Source: CAD feature listing. Evaluate the final solid. Frame: model axes, mm. A direction names the side the tool comes from. Give positions to 0.01 mm unless a question says otherwise; leave off trailing zeros. Write each loop counter-clockwise with the first axis right and the second up, starting at its lowest first coordinate (ties: lowest second). Pieces come first, ordered by that corner, then holes. Notation, with made-up numbers: (-28, 63.25) -> (20, 63.25) arc R29 cw to (20, 85.25) -> close; hole circle Ø1 at (89.25, -7.75). An arc over 180 degrees is marked (long way). Answer as a JSON object with one key per item and string values. Group by question number.
Item 1: Pull-direction query (X, two-part tool) for faces 1 (the face through (18.01, 9.86, -72.15)), 2 (the face through (27, 5, -103)), 3 (the face through (9, 10, 0)); classes: pulls with the +X half, pulls with the -X half, needs draft (parallel to the pull), parting line crosses it, or undercut.
Item 2: Section query B-B on z = -28. Return the cut outline in (x, y), plus the area to 3 significant figures.
Item 3: Section query D-D on z = -97. Return the cut outline in (x, y).
Item 4: Section query A-A on y = 8. Return the cut outline in (x, z).
Item 5: Ray query, probe 1 along X at (y, z) = (16, -26); probe 2 along Z at (x, y) = (31, 5.5); probe 3 along Z at (x, y) = (6.5, 7). Return the intervals inside material, ascending. Write a range as from..to.
Item 6: Access query for faces 4 (the face through (15.57, 9.86, -5.6)), 5 (the face through (33, 20, -76)), 6 (the face through (19.43, 9.86, -0.6)), 7 (the face through (33, 16.899, -96)). Directions: +Z, -Z, +X, -X, +Y, -Y. A direction counts if a zero-diameter tool reaches every point of the face in a straight line with its end or side. Return the directions, or none.
Item 7: Section query C-C on y = -3.5. Return the cut outline in (x, z), plus the area to 3 significant figures.
Item 8: First-contact query: pin 1 Ø17.5 at (y, z) = (-5.5, -101) entering from +X; pin 2 Ø12 at (x, z) = (19.5, -18) entering from -Y; pin 3 Ø3.5 at (x, z) = (34, -95.5) entering from -Y; pin 4 Ø3 at (x, z) = (23.5, -72) entering from +Y. Flat tips, straight axial feed; report the tip coordinate or a pass-through.
from build123d import *

# Parameters (mm, degrees)
EXTRUDE_1_DEPTH     = 20
EXTRUDE_2_DEPTH     = 64
CUT_EXTRUDE_1_DEPTH = 64


with BuildPart() as part:
    # Эскиз4 → Бобышка-Вытянуть1 (new body)
    with BuildSketch(Plane(origin=(0, 0, 0), x_dir=(1, 0, 0), z_dir=(0, 1, 0))):
        with BuildLine():
            Line((0, 0), (0, 90))
            Line((0, 90), (65, 90))
            Line((65, 90), (65, 0))
            Line((65, 0), (47, 0))
            ThreePointArc((47, 0), (45.585786438, 0.585786438), (45, 2))
            Line((45, 2), (45, 3))
            ThreePointArc((45, 3), (45.585786438, 4.414213562), (47, 5))
            Line((47, 5), (48, 5))
            ThreePointArc((48, 5), (49.414213562, 5.585786438), (50, 7))
            Line((50, 7), (50, 65))
            ThreePointArc((50, 65), (47.071067812, 72.071067812), (40, 75))
            Line((40, 75), (25, 75))
            ThreePointArc((25, 75), (17.928932188, 72.071067812), (15, 65))
            Line((15, 65), (15, 7))
            ThreePointArc((15, 7), (15.585786438, 5.585786438), (17, 5))
            Line((17, 5), (18, 5))
            ThreePointArc((18, 5), (19.414213562, 4.414213562), (20, 3))
            Line((20, 3), (20, 2))
            ThreePointArc((20, 2), (19.414213562, 0.585786438), (18, 0))
            Line((18, 0), (0, 0))
        make_face()
    extrude(amount=EXTRUDE_1_DEPTH)

    # Эскиз6 → Бобышка-Вытянуть2 (add)
    with BuildSketch(Plane(origin=(65, 0, 0), x_dir=(0, 0, -1), z_dir=(1, 0, 0))):
        Polygon((90, 20), (106, 20), (106, -20), (102, -20), (102, 16.898771426), (90, 16.898771426), align=None)
    extrude(amount=-EXTRUDE_2_DEPTH)

    # Эскиз7 → Вырез-Вытянуть1 (cut)
    with BuildSketch(Plane(origin=(0, 20, 0), x_dir=(1, 0, 0), z_dir=(0, 1, 0))):
        Polygon((27, 109.944844375), (27, 90), (-10.963229583, 90), (-10.963229583, 111.789211804), align=None)
        Polygon((39, 90), (39, 113.326184662), (82.188937299, 109.944844375), (82.188937299, 90), align=None)
    extrude(amount=-CUT_EXTRUDE_1_DEPTH, mode=Mode.SUBTRACT)


solid = part.part
Worked answers:
{
 "1": {"face 1": "undercut", "face 2": "pulls with the -X half", "face 3": "needs draft"},
 "2": {"outline": "(0, 0) -> (15, 0) -> (15, 20) -> (0, 20) -> close; (50, 0) -> (65, 0) -> (65, 20) -> (50, 20) -> close", "area": "600 mm^2"},
 "3": {"outline": "(27, 16.9) -> (39, 16.9) -> (39, 20) -> (27, 20) -> close"},
 "4": {"outline": "(0, -90) -> (65, -90) -> (65, 0) -> (47, 0) arc R2 ccw to (45, -2) -> (45, -3) arc R2 ccw to (47, -5) -> (48, -5) arc R2 cw to (50, -7) -> (50, -65) arc R10 cw to (40, -75) -> (25, -75) arc R10 cw to (15, -65) -> (15, -7) arc R2 cw to (17, -5) -> (18, -5) arc R2 ccw to (20, -3) -> (20, -2) arc R2 ccw to (18, 0) -> (0, 0) -> close; (27, -106) -> (39, -106) -> (39, -102) -> (27, -102) -> close"},
 "5": {"probe 1": "0..15, 50..65", "probe 2": "-106..-102, -90..-75", "probe 3": "-90..0"},
 "6": {"face 4": "+Y, -Y", "face 5": "+Z, -Z, +X, -X, +Y", "face 6": "+Z, +Y, -Y", "face 7": "+X, -X, -Y"},
 "7": {"outline": "(27, -106) -> (39, -106) -> (39, -102) -> (27, -102) -> close", "area": "48.0 mm^2"},
 "8": {"pin 1": "x = 39", "pin 2": "y = 0", "pin 3": "y = 16.9", "pin 4": "through"}
}
